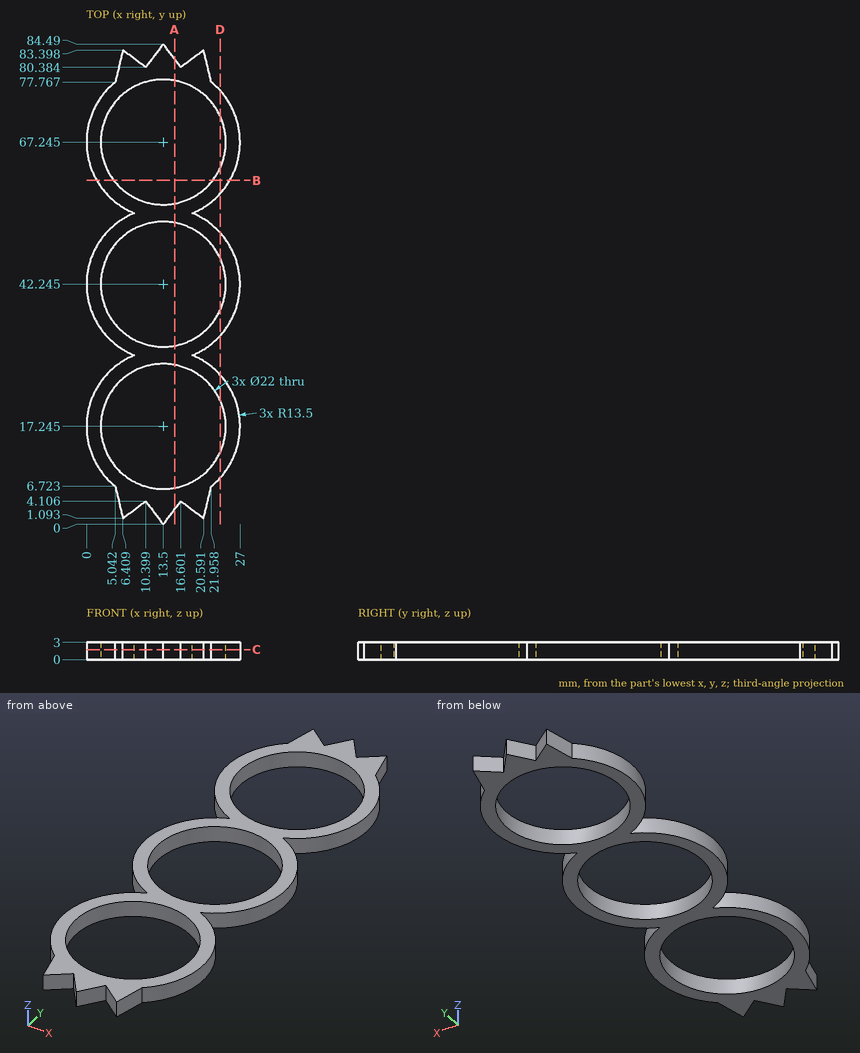
Geometry: see drawing. Coordinates: mm, zero at the bounding-box minimum. Give positions to 0.01 mm unless a question says otherwise; leave off trailing zeros. Loops run counter-clockwise (first coordinate to the right, second up) from the corner with the lowest first, then second, coordinate; pieces in that order, holes last. Notation, with made-up numbers: (87, -12.75) -> (120, -12.75) arc R24 cw to (120, 14.25) -> close; hole circle Ø4 at (49.5, -12.75). An arc over 180 degrees is marked (long way). Use CSV: the item, a comma, the result in double quotes.
(1) Cut plane C-C (z = 1.75). Output: boundary loops of the cut face in (x, y) (1 decimal).
From the geometry:
outline,"(5, 6.7) -> (6.4, 1.1) -> (10.4, 4.1) -> (13.5, 0) -> (16.6, 4.1) -> (20.6, 1.1) -> (22, 6.7) arc R13.5 ccw to (18.6, 29.7) arc R13.5 ccw to (18.6, 54.7) arc R13.5 ccw to (22, 77.8) -> (20.6, 83.4) -> (16.6, 80.4) -> (13.5, 84.5) -> (10.4, 80.4) -> (6.4, 83.4) -> (5, 77.8) arc R13.5 ccw to (8.4, 54.7) arc R13.5 ccw to (8.4, 29.7) arc R13.5 ccw to start; hole circle Ø22 at (13.5, 17.2); hole circle Ø22 at (13.5, 42.2); hole circle Ø22 at (13.5, 67.2)"
(2) Cut plane B-B (y = 60.5). Output: boundary loops of the cut face in (x, z) (1 decimal).
From the geometry:
outline,"(1.8, 0) -> (4.8, 0) -> (4.8, 3) -> (1.8, 3) -> close; (22.2, 0) -> (25.2, 0) -> (25.2, 3) -> (22.2, 3) -> close"
(3) Ray query, line 1 along Y through (x, z) = (14.25, 2.8) (1 decimal); line 2 along X through (y, z) = (18, 1.5) (1 decimal); line 3 along Y through (x, z) = (22.5, 2) (1 decimal). Return the intervals inside material, ascending. Write a range as [from, to].
From the geometry:
line 1,"[1, 6.3], [28.2, 31.3], [53.2, 56.3], [78.2, 83.5]"
line 2,"[0, 2.5], [24.5, 27]"
line 3,"[7.2, 10.9], [23.6, 27.3], [32.2, 35.9], [48.6, 52.3], [57.2, 60.9], [73.6, 77.3]"
(4) Cut plane A-A (x = 15.5). Output: boundary loops of the cut face in (y, z).
From the geometry:
outline,"(2.65, 0) -> (6.43, 0) -> (6.43, 3) -> (2.65, 3) -> close; (28.06, 0) -> (31.43, 0) -> (31.43, 3) -> (28.06, 3) -> close; (53.06, 0) -> (56.43, 0) -> (56.43, 3) -> (53.06, 3) -> close; (78.06, 0) -> (81.84, 0) -> (81.84, 3) -> (78.06, 3) -> close"
(5) First-contact query: P1, Ø1, axis at y = 64, z = 0.5, coming from the -X side; P2, Ø1.5, axis at y = 55, z = 1, coming from the -X side; P3, Ø13, axis at x = 13.5, y = 67.25, coming from the +Z side. Flat tips, straight axial feed; report the tip coordinate or a pass-through.
From the geometry:
P1,"x = 0.28"
P2,"x = 6.42"
P3,"through"
(6) Cut plane D-D (x = 23.5). Output: boundary loops of the cut face in (y, z) (1 decimal).
From the geometry:
outline,"(8.2, 0) -> (12.7, 0) -> (12.7, 3) -> (8.2, 3) -> close; (21.8, 0) -> (26.3, 0) -> (26.3, 3) -> (21.8, 3) -> close; (33.2, 0) -> (37.7, 0) -> (37.7, 3) -> (33.2, 3) -> close; (46.8, 0) -> (51.3, 0) -> (51.3, 3) -> (46.8, 3) -> close; (58.2, 0) -> (62.7, 0) -> (62.7, 3) -> (58.2, 3) -> close; (71.8, 0) -> (76.3, 0) -> (76.3, 3) -> (71.8, 3) -> close"
